Design review of the part shown in the three views and the two pictorial views. Dimensions are in mm from the part's minimum x, y and z. A direction names the side the tool comes from. Coordinates: 2 decimals unless noted, no trailing zeros. Loops run counter-clockwise (first coordinate to the right, second up) from the corner with the lowest first, then second, coordinate; pieces in that order, holes last.
Q1. For P1, Ø3.5, axis at y = 39, z = 5, coming from the -X side; P2, Ø2, axis at x = 7.5, z = 2, coming from the +Y side; P3, Ø2, axis at x = 13, z = 5, coming from the +Y side; P4, Ø1.5, axis at x = 22, y = 15.5, coming from the +Z side, all flat-tipped, find the tip position at first contact; note any pin that passes through.
Q2. Wall thickness on probe 1 along X at (y, z) = (5, 9); probe 2 along Z at (x, y) = (24.65, 39); probe 3 along Y at (x, z) = (18.5, 4.5): over which ranges is each line inside the solid? List them lowest first.
Q3. Draft analysis for pull direction X (two halves, no side actions). For the marked faces 1, 2, 3 and 4, state which applies: released by +X, released by -X, zero draft, split by the parting line, or undercut.
Q4. Add section C-C on x = 25.5. Give the boundary of the cut face in (y, z), and give its area (3 significant figures).
Q5. Add section B-B on y = 39. Give the boundary of the cut face in (x, z).
Q6. Add section D-D on y = 10. Give the boundary of the cut face in (x, z).
Q7. Add section A-A on z = 5. Give the boundary of the cut face in (x, y), and give its area (3 significant figures).
Q8. Machinability: for the marked faces 5, 6 and 7, which of the approach directions +Z, -Z, +X, -X, +Y, -Y give a long, thin tool a straight path to every point of the face, cutting with its end or side? Answer none if there is none.
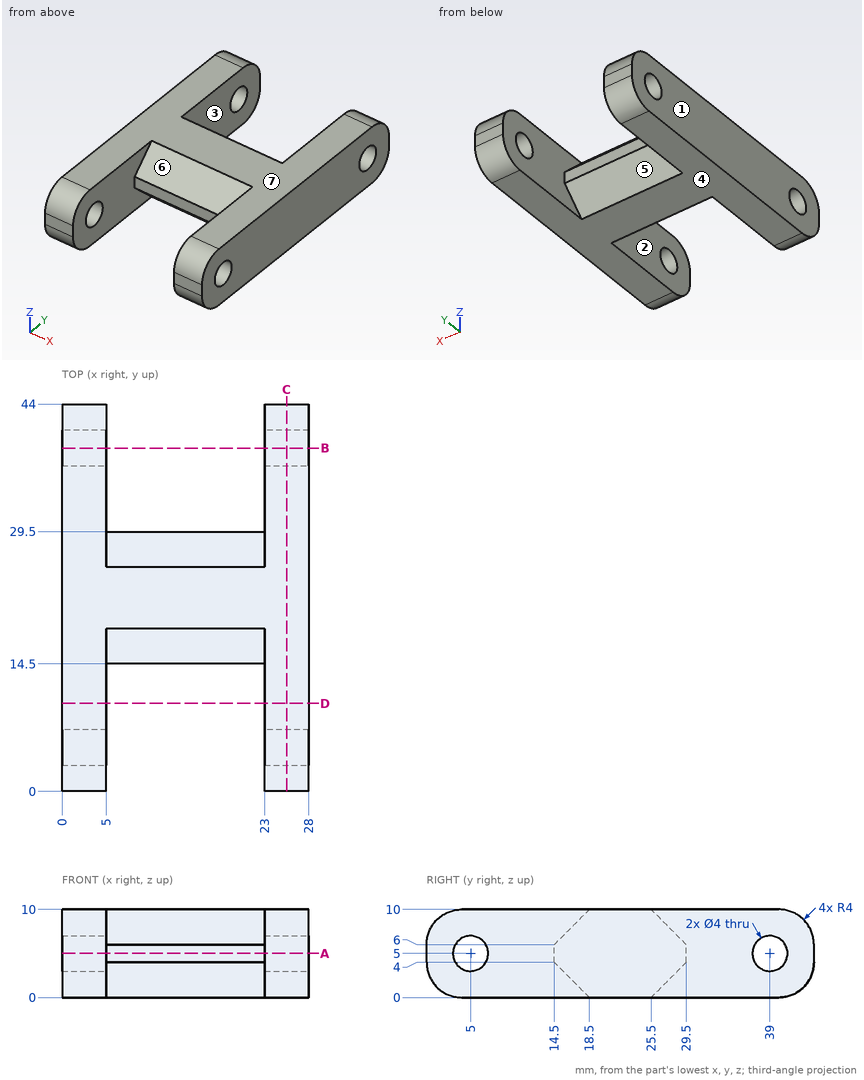
Entries:
1. P1: passes through
1. P2: stops at y = 28.5
1. P3: stops at y = 29.5
1. P4: stops at z = 7.75
2. probe 1: x = 0 to 5, 23 to 28
2. probe 2: z = 0 to 3, 7 to 10
2. probe 3: y = 14.5 to 29.5
3. face 1: released by -X
3. face 2: undercut
3. face 3: undercut
3. face 4: zero draft
4. outline: (0, 4) arc R4 ccw to (4, 0) - (40, 0) arc R4 ccw to (44, 4) - (44, 6) arc R4 ccw to (40, 10) - (4, 10) arc R4 ccw to (0, 6) - close; hole circle Ø4 at (5, 5); hole circle Ø4 at (39, 5)
4. area: 401 mm2
5. outline: (0, 0) - (5, 0) - (5, 3) - (0, 3) - close; (0, 7) - (5, 7) - (5, 10) - (0, 10) - close; (23, 0) - (28, 0) - (28, 3) - (23, 3) - close; (23, 7) - (28, 7) - (28, 10) - (23, 10) - close
6. outline: (0, 0) - (5, 0) - (5, 10) - (0, 10) - close; (23, 0) - (28, 0) - (28, 10) - (23, 10) - close
7. outline: (0, 0) - (5, 0) - (5, 3) - (0, 3) - close; (0, 7) - (5, 7) - (5, 14.5) - (23, 14.5) - (23, 7) - (28, 7) - (28, 37) - (23, 37) - (23, 29.5) - (5, 29.5) - (5, 37) - (0, 37) - close; (0, 41) - (5, 41) - (5, 44) - (0, 44) - close; (23, 0) - (28, 0) - (28, 3) - (23, 3) - close; (23, 41) - (28, 41) - (28, 44) - (23, 44) - close
7. area: 630 mm2
8. face 5: -Z, +Y
8. face 6: +Z, -Y
8. face 7: +Z, +X, -X, +Y, -Y
